Autodesk Inventor part; units mm, degrees
ref_plane "YZ Plane" through (0, 0, 0) normal (1, 0, 0) x (0, 1, 0)
ref_plane "XZ Plane" through (0, 0, 0) normal (0, 1, 0) x (-1, 0, 0)
ref_plane "XY Plane" through (0, 0, 0) normal (0, 0, 1) x (1, 0, 0)
sketch "Sketch1" plane through (0, 0, 0) normal (0, 0, 1) x (1, 0, 0)
  circle A0 centre (0, 0) radius 25
  circle A1 centre (40, 48.6) radius 25
  circle A2 centre (-40, 48.6) radius 25
  line L0 (-40, 73.6) -> (40, 73.6)
  line L1 (59.3028, 32.7129) -> (19.3028, -15.8871)
  line L2 (-19.3028, -15.8871) -> (-59.3028, 32.7129)
  dimension "d0" = 50
  dimension "d1" = 50
  dimension "d2" = 50
  dimension "d3" = 40
  dimension "d4" = 40
  dimension "d5" = 48.6
  dimension "d6" = 48.6
extrude "Extrusion1" add sketch "Sketch1" along normal blind 10
sketch "Sketch2" plane through (0, 0, 10) normal (0, 0, 1) x (1, 0, 0)
  arc A0 (-40, 73.6) -> (-59.3028, 32.7129) centre (-40, 48.6) ccw
  line L0 (-59.3028, 32.7129) -> (-19.3028, -15.8871)
  arc A1 (-19.3028, -15.8871) -> (19.3028, -15.8871) centre (0, 0) ccw
  line L1 (19.3028, -15.8871) -> (59.3028, 32.7129)
  arc A2 (59.3028, 32.7129) -> (40, 73.6) centre (40, 48.6) ccw
  line L2 (40, 73.6) -> (-40, 73.6)
  circle A3 centre (40, 48.6) radius 2.5
  circle A4 centre (0, 0) radius 2.5
  circle A5 centre (-40, 48.6) radius 2.5
  dimension "d10" = 5
  dimension "d11" = 5
  dimension "d12" = 5
extrude "Extrusion2" cut sketch "Sketch2" against normal up to next contours A3 | A4 | A5
sketch "Sketch3" plane through (0, 0, 10) normal (0, 0, 1) x (1, 0, 0)
  circle A0 centre (-15, 58.6) radius 2.5
  circle A1 centre (15, 58.6) radius 2.5
  circle A2 centre (-15, 28.6) radius 2.5
  circle A3 centre (15, 28.6) radius 2.5
  circle A4 centre (0, 0) radius 2.5
  circle A5 centre (40, 48.6) radius 2.5
  circle A6 centre (-40, 48.6) radius 2.5
  arc A7 (-40, 73.6) -> (-59.3028, 32.7129) centre (-40, 48.6) ccw
  line L0 (-59.3028, 32.7129) -> (-19.3028, -15.8871)
  arc A8 (-19.3028, -15.8871) -> (19.3028, -15.8871) centre (0, 0) ccw
  line L1 (19.3028, -15.8871) -> (59.3028, 32.7129)
  arc A9 (59.3028, 32.7129) -> (40, 73.6) centre (40, 48.6) ccw
  line L2 (40, 73.6) -> (-40, 73.6)
  dimension "d15" = 5
  dimension "d16" = 5
  dimension "d17" = 5
  dimension "d18" = 5
  dimension "d19" = 30
  dimension "d20" = 30
  dimension "d21" = 30
  dimension "d22" = 30
  dimension "d23" = 15
  dimension "d24" = 15
  dimension "d25" = 15
  dimension "d26" = 15
extrude "Extrusion3" cut sketch "Sketch3" against normal up to next contours A0 | A1 | A2 | A3
properties part number "Arm_Base-SquareBar-Rev3-2" material "Bronze, Cast"
Here's how the part is built. I have some questions about the finished solid (model axes, mm). Coordinates: 2 decimals unless noted, no trailing zeros. Order: outer loops, then holes, each group sorted by start corner. A loop starts at its lowest first (then second) coordinate and runs counter-clockwise, first axis right, second up. Notation, with made-up numbers: (0, -9.5) - (57, -9.5) arc R32 cw to (57, 17.5) - close; hole circle Ø3 at (50.25, 77.25). An arc over 180 degrees is marked (long way). One line per question, with ' | ' between items. Start each with the question number.
1. Please list where these lines run through material, in increasing order: line 1 along Y through (x, z) = (0, 6); line 2 along Y through (x, z) = (-15, 6.25); line 3 along X through (y, z) = (59, 1.5). Write a range as [from, to].
2. If we section it at B-B (y = 28.6): Write out the boundary of the cut face in (x, z).
3. If we section it at D-D (z = 2.75): Write out the boundary of the cut face in (x, y), and give its area (3 significant figures).
4. If we section it at C-C (y = 0): Write out the boundary of the cut face in (x, z).
5. If we mould it in two halves opening along X, with no side actions, what happens to faces 1 (the cylindrical face through (-16.84, 60.29, 5.07)), 2 (the flat face through (-1, 36, 0)), 3 (the cylindrical face through (-62.773, 58.914, 4.93))? For each: released by +X, released by -X, zero draft, split by the parting line, or undercut.
6. If we section it at A-A (x = -15): Write out the boundary of the cut face in (y, z).
7. I'm going to push flat-ended pins straight in: pin 1 Ø4 at (y, z) = (56, 6.5) entering from -X; pin 2 Ø5 at (x, z) = (-15, 8) entering from -Y; pin 3 Ø1 at (x, z) = (-3.5, 8) entering from -Y. Where does each tip first touch, or does it pass through?
Model answer:
1) line 1: y = [-25, -2.5], [2.5, 73.6] | line 2: y = [-20, 26.1], [31.1, 56.1], [61.1, 73.6] | line 3: x = [-62.73, -17.47], [-12.53, 12.53], [17.47, 62.73]
2) outline: (-55.92, 0) - (-17.5, 0) - (-17.5, 10) - (-55.92, 10) - close; (-12.5, 0) - (12.5, 0) - (12.5, 10) - (-12.5, 10) - close; (17.5, 0) - (55.92, 0) - (55.92, 10) - (17.5, 10) - close
3) outline: (-59.3, 32.71) - (-19.3, -15.89) arc R25 ccw to (19.3, -15.89) - (59.3, 32.71) arc R25 ccw to (40, 73.6) - (-40, 73.6) arc R25 ccw to start; hole circle Ø5 at (-40, 48.6); hole circle Ø5 at (-15, 28.6); hole circle Ø5 at (-15, 58.6); hole circle Ø5 at (0, 0); hole circle Ø5 at (15, 28.6); hole circle Ø5 at (15, 58.6); hole circle Ø5 at (40, 48.6) | area: 8,920 mm²
4) outline: (-32.38, 0) - (-2.5, 0) - (-2.5, 10) - (-32.38, 10) - close; (2.5, 0) - (32.38, 0) - (32.38, 10) - (2.5, 10) - close
5) face 1: undercut | face 2: zero draft | face 3: released by -X
6) outline: (-20, 0) - (26.1, 0) - (26.1, 10) - (-20, 10) - close; (31.1, 0) - (56.1, 0) - (56.1, 10) - (31.1, 10) - close; (61.1, 0) - (73.6, 0) - (73.6, 10) - (61.1, 10) - close
7) pin 1: stops at x = -64.41 | pin 2: stops at y = -21.65 | pin 3: stops at y = -24.82
